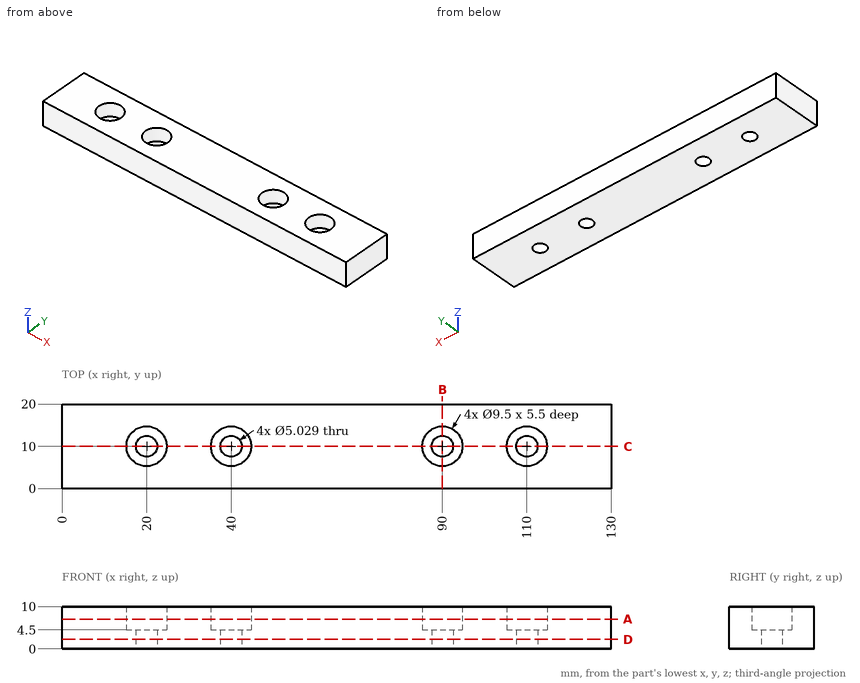
Job drawing, mm, ordinate dimensions from the low corner. One solid piece. Give positions to 0.01 mm unless a question says otherwise; leave off trailing zeros. Loops run counter-clockwise (first coordinate to the right, second up) from the corner with the lowest first, then second, coordinate; pieces in that order, holes last. Notation, with made-up numbers: (56, -4.5) -> (102, -4.5) arc R19 cw to (102, 10.5) -> close; hole circle Ø2 at (22, 16). An arc over 180 degrees is marked (long way). Use a Markdown table: item, result. Add a question column.
(1) Slice it at C-C on y = 10. Give the number of separate pieces and of enclosed holes in the cut face, and give its area (3 significant figures).
(2) Slice it at B-B on x = 90. List the corners of the cut face in (y, z).
(3) Slice it at D-D on z = 2.25. List the corners of the cut face in (x, y), and give its area (3 significant figures).
(4) Drop flat-ended pins along their axis: pin 1 Ø2 at (x, y) = (18, 7.5) entering from +Z; pin 2 Ø6 at (y, z) = (16.5, 2) entering from -X. Give the stop position or say it passes through.
(5) Wall check: line 1 along X through (y, z) = (10, 9.5); line 2 along X through (y, z) = (10, 3.4); line 3 along Y through (x, z) = (40, 3.05). Give the ranges that are in metal, low to high.
(6) Slice it at A-A on z = 7. List the corners of the cut face in (x, y).
Filled sheet:
| question | item | result |
|---|---|---|
| 1 | separate pieces | 5 |
| 1 | enclosed holes | 0 |
| 1 | area | 1,000 mm2 |
| 2 | outline | (0, 0) -> (7.49, 0) -> (7.49, 4.5) -> (5.25, 4.5) -> (5.25, 10) -> (0, 10) -> close; (12.51, 0) -> (20, 0) -> (20, 10) -> (14.75, 10) -> (14.75, 4.5) -> (12.51, 4.5) -> close |
| 3 | outline | (0, 0) -> (130, 0) -> (130, 20) -> (0, 20) -> close; hole circle Ø5.03 at (20, 10); hole circle Ø5.03 at (40, 10); hole circle Ø5.03 at (90, 10); hole circle Ø5.03 at (110, 10) |
| 3 | area | 2,520 mm2 |
| 4 | pin 1 | z = 4.5 |
| 4 | pin 2 | x = 0 |
| 5 | line 1 | 0 to 15.25, 24.75 to 35.25, 44.75 to 85.25, 94.75 to 105.25, 114.75 to 130 |
| 5 | line 2 | 0 to 17.49, 22.51 to 37.49, 42.51 to 87.49, 92.51 to 107.49, 112.51 to 130 |
| 5 | line 3 | 0 to 7.49, 12.51 to 20 |
| 6 | outline | (0, 0) -> (130, 0) -> (130, 20) -> (0, 20) -> close; hole circle Ø9.5 at (20, 10); hole circle Ø9.5 at (40, 10); hole circle Ø9.5 at (90, 10); hole circle Ø9.5 at (110, 10) |
